The listing builds one solid part. Answer for the finished solid, in the listing's coordinates (mm). A direction names the side the tool comes from. Give positions to 0.01 mm unless a question says otherwise; leave off trailing zeros. Order: outer loops, then holes, each group sorted by start corner. A loop starts at its lowest first (then second) coordinate and runs counter-clockwise, first axis right, second up.
```python
from build123d import *

# Parameters (mm, degrees)
F0_W     = 304.8
F0_H     = 304.8
F1_DEPTH = 25.4
F2_W     = 304.8
F2_H     = 330.2
F3_DEPTH = 25.4
F5_W     = 355.6
F5_H     = 330.2
F6_DEPTH = 25.4
F7_W     = 355.6
F7_H     = 330.2
F8_DEPTH = 25.4


with BuildPart() as f1:
    # F0 (on Top) → F1 (new body)
    with BuildSketch(Plane.XY):
        Rectangle(F0_W, F0_H)
    extrude(amount=F1_DEPTH)

    # F2 (on face) → F3 (join)
    with BuildSketch(Plane.XZ.offset(152.4)):
        with Locations((0, 165.1)):
            Rectangle(F2_W, F2_H)
    extrude(amount=F3_DEPTH)

    # F4: F1 across plane


with BuildPart() as f1_1:
    add(f1.part)
    add(f1.part.mirror(Plane.XZ))

    # F5 (on face) → F6 (join)
    with BuildSketch(Plane(origin=(-152.4, 0, 0), x_dir=(0, -1, 0), z_dir=(-1, 0, 0))):
        with Locations((0, 165.1)):
            Rectangle(F5_W, F5_H)
    extrude(amount=F6_DEPTH)

    # F7 (on face) → F8 (join)
    with BuildSketch(Plane.YZ.offset(152.4)):
        with Locations((0, 165.1)):
            Rectangle(F7_W, F7_H)
    extrude(amount=F8_DEPTH)


solid = f1_1.part
```
1) Find section A-A (z = 99.5). Write down the section's boundary in (x, y), then the cut area to 3 significant figures.
Geometry says:
outline: (-177.8, -177.8) - (177.8, -177.8) - (177.8, 177.8) - (-177.8, 177.8) - close; hole (-152.4, -152.4) - (152.4, -152.4) - (152.4, 152.4) - (-152.4, 152.4) - close
area: 33,500 mm2
2) Straight lines are drawn through the part: probe 1 along X at (y, z) = (-52, 73.5); probe 2 along Z at (x, y) = (7.5, 97). For each, find the intervals that lie inside material, in ascending order.
Geometry says:
probe 1: x = -177.8 to -152.4, 152.4 to 177.8
probe 2: z = 0 to 25.4
3) Given P1, Ø1.5, axis at x = 116.5, y = -17, coming from the +Z side, flat-ended and moving along its own axis, determine where the tip first touches the part or whether it passes through.
Geometry says:
P1: stops at z = 25.4
4) For a pull along Y with two mould halves and no side action, classify faces 1 (the flat face through (-2, 156, 330.2)), 2 (the flat face through (-2, 177.8, 163)), 3 (the flat face through (-2, 2, 25.4)) as +Y half, -Y half, draft (parallel to the pull), parting line (faces both ways), or undercut.
Geometry says:
face 1: draft
face 2: +Y half
face 3: undercut
5) Find section B-B (x = 77). Write down the section's boundary in (y, z).
Geometry says:
outline: (-177.8, 0) - (177.8, 0) - (177.8, 330.2) - (152.4, 330.2) - (152.4, 25.4) - (-152.4, 25.4) - (-152.4, 330.2) - (-177.8, 330.2) - close
6) A tool of negligible diameter and unlimited length cuts with its end or side. For faces 4 (the flat face through (-152.4, 2, 180)), 5 (the flat face through (-2, -177.8, 163)), from which of +Z, -Z, +X, -X, +Y, -Y can it reach the whole face along a straight path? Write none if from no direction.
Geometry says:
face 4: +Z
face 5: +Z, -Z, +X, -X, -Y
